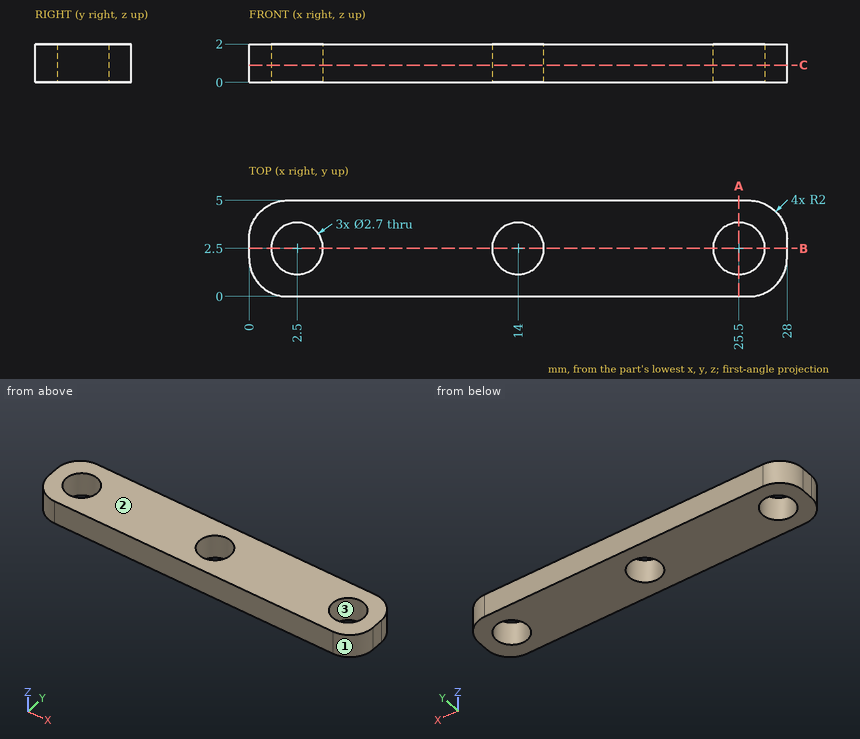
Geometry: see drawing. Coordinates: mm, zero at the bounding-box minimum. Coordinates: 2 decimals unless noted, no trailing zeros. Loops run counter-clockwise (first coordinate to the right, second up) from the corner with the lowest first, then second, coordinate; pieces in that order, holes last. Notation, with made-up numbers: (7.25, -23.75) - (65.25, -23.75) arc R14 cw to (65.25, -19.75) - close; hole circle Ø11 at (-29.5, 18). An arc over 180 degrees is marked (long way). Answer in a Markdown table with one row per item.
(1) Material intervals for L1, parallel to X at y = 3.7, z = 1.25; L2, parallel to X at y = 2.65, z = 0.2; L3, parallel to Y at x = 25.5, z = 1.55, sorted ascending. Write a range as from..to.
Model answer:
| item | result |
|---|---|
| L1 | x = 0.13..1.88, 3.12..13.38, 14.62..24.88, 26.12..27.87 |
| L2 | x = 0..1.16, 3.84..12.66, 15.34..24.16, 26.84..28 |
| L3 | y = 0..1.15, 3.85..5 |
(2) Cut plane A-A on x = 25.5. Output: boundary loops of the cut face in (y, z).
Model answer:
| item | result |
|---|---|
| outline | (0, 0) - (1.15, 0) - (1.15, 2) - (0, 2) - close; (3.85, 0) - (5, 0) - (5, 2) - (3.85, 2) - close |
(3) Pin query (flat end, axial travel): P1, Ø2, axis at x = 14, y = 2.5, coming from the +Z side; P2, Ø1, axis at y = 1, z = 0.5, coming from the -X side. Return the tip coordinate at first contact, or that it passes through.
Model answer:
| item | result |
|---|---|
| P1 | passes through |
| P2 | stops at x = 0.06 |
(4) Cut plane B-B on y = 2.5. Output: boundary loops of the cut face in (x, z).
Model answer:
| item | result |
|---|---|
| outline | (0, 0) - (1.15, 0) - (1.15, 2) - (0, 2) - close; (3.85, 0) - (12.65, 0) - (12.65, 2) - (3.85, 2) - close; (15.35, 0) - (24.15, 0) - (24.15, 2) - (15.35, 2) - close; (26.85, 0) - (28, 0) - (28, 2) - (26.85, 2) - close |
(5) Cut plane C-C on z = 0.9. Output: boundary loops of the cut face in (x, y), plus the area to 3 significant figures.
Model answer:
| item | result |
|---|---|
| outline | (0, 2) arc R2 ccw to (2, 0) - (26, 0) arc R2 ccw to (28, 2) - (28, 3) arc R2 ccw to (26, 5) - (2, 5) arc R2 ccw to (0, 3) - close; hole circle Ø2.7 at (2.5, 2.5); hole circle Ø2.7 at (14, 2.5); hole circle Ø2.7 at (25.5, 2.5) |
| area | 119 mm² |
(6) Mould query, pull axis X, two halves, no side actions, for the marked faces 1, 2 and 3. Classes: pulls with the +X half, pulls with the -X half, needs draft (parallel to the pull), parting line crosses it, or undercut.
Model answer:
| item | result |
|---|---|
| face 1 | pulls with the +X half |
| face 2 | needs draft |
| face 3 | undercut |
